Could you check a few things on this model? Use its own coordinates, in mm. A direction names the side the tool comes from. Give positions to 0.01 mm unless a question says otherwise; leave off trailing zeros. Loops run counter-clockwise (first coordinate to the right, second up) from the corner with the lowest first, then second, coordinate; pieces in that order, holes last. Notation, with made-up numbers: (75.25, -31) - (89.25, -31) arc R6 cw to (89.25, -23) - close; hole circle Ø9 at (48.25, 50). An arc over 180 degrees is marked (long way). Write each question's results on one line, items separated by ' | '. Start each with the question number.
```python
from build123d import *

# Parameters (mm, degrees)
SKETCH1_W           = 8.5
SKETCH1_H           = 8.5
BOSS_EXTRUDE1_DEPTH = 5
SKETCH2_W           = 8.5
SKETCH2_H           = 8.5
BOSS_EXTRUDE2_DEPTH = 2
SKETCH3_R           = 1.5
CUT_EXTRUDE1_DEPTH  = 2
SKETCH4_W           = 80
SKETCH4_H           = 8.5
BOSS_EXTRUDE3_DEPTH = 3
SKETCH5_W           = 7
SKETCH5_H           = 8.5
BOSS_EXTRUDE4_DEPTH = 8.5
CUT_EXTRUDE2_DEPTH  = 5
SKETCH7_R           = 1.5
CUT_EXTRUDE3_DEPTH  = 5
CUT_EXTRUDE4_DEPTH  = 10
SKETCH9_W           = 8.5
SKETCH9_H           = 8.5
SKETCH9_R           = 1.5
BOSS_EXTRUDE5_DEPTH = 2
CUT_EXTRUDE5_DEPTH  = 2
SKETCH11_W          = 8.5
SKETCH11_H          = 8.5
SKETCH11_R          = 1.5
BOSS_EXTRUDE6_DEPTH = 2
BOSS_EXTRUDE7_DEPTH = 5
BOSS_EXTRUDE8_DEPTH = 5
SKETCH14_W          = 8.5
SKETCH14_H          = 11.5
CUT_EXTRUDE6_DEPTH  = 4
SKETCH15_W          = 8.5
SKETCH15_H          = 11.5
CUT_EXTRUDE7_DEPTH  = 4
SKETCH16_R          = 1.5
CUT_EXTRUDE8_DEPTH  = 4
SKETCH17_R          = 1.5
CUT_EXTRUDE9_DEPTH  = 4


with BuildPart() as part:
    # Sketch1 → Boss-Extrude1 (new body)
    with BuildSketch(Plane(origin=(0, 0, 0), x_dir=(0, 0, -1), z_dir=(1, 0, 0))):
        Rectangle(SKETCH1_W, SKETCH1_H)
        Polygon((1.58771324, 2.75), (-1.58771324, 2.75), (-3.175426481, 0), (-1.58771324, -2.75), (1.58771324, -2.75), (3.175426481, 0), align=None, mode=Mode.SUBTRACT)
    extrude(amount=BOSS_EXTRUDE1_DEPTH)

    # Sketch2 → Boss-Extrude2 (add)
    with BuildSketch(Plane.ZY):
        Rectangle(SKETCH2_W, SKETCH2_H)
    extrude(amount=BOSS_EXTRUDE2_DEPTH)

    # Sketch3 → Cut-Extrude1 (cut)
    with BuildSketch(Plane(origin=(0, 0, 0), x_dir=(0, 0, -1), z_dir=(1, 0, 0))):
        Circle(SKETCH3_R)
    extrude(amount=-CUT_EXTRUDE1_DEPTH, mode=Mode.SUBTRACT)

    # Sketch4 → Boss-Extrude3 (add)
    with BuildSketch(Plane.XZ.offset(4.25)):
        with Locations((38, 0)):
            Rectangle(SKETCH4_W, SKETCH4_H)
    extrude(amount=BOSS_EXTRUDE3_DEPTH)

    # Sketch5 → Boss-Extrude4 (add)
    with BuildSketch(Plane(origin=(0, -4.25, 0), x_dir=(1, 0, 0), z_dir=(0, 1, 0))):
        with Locations((74.5, 0)):
            Rectangle(SKETCH5_W, SKETCH5_H)
    extrude(amount=BOSS_EXTRUDE4_DEPTH)

    # Sketch6 → Cut-Extrude2 (cut)
    with BuildSketch(Plane.ZY.offset(-71)):
        Polygon((3.175426481, 0), (1.58771324, 2.75), (-1.58771324, 2.75), (-3.175426481, 0), (-1.58771324, -2.75), (1.58771324, -2.75), align=None)
    extrude(amount=-CUT_EXTRUDE2_DEPTH, mode=Mode.SUBTRACT)

    # Sketch7 → Cut-Extrude3 (cut)
    with BuildSketch(Plane.ZY.offset(-76)):
        Circle(SKETCH7_R)
    extrude(amount=-CUT_EXTRUDE3_DEPTH, mode=Mode.SUBTRACT)

    # Sketch8 → Cut-Extrude4 (cut)
    with BuildSketch(Plane.ZY.offset(2)):
        Polygon((-1.58771324, 2.75), (1.58771324, 2.75), (3.175426481, 0), (1.58771324, -2.75), (-1.58771324, -2.75), (-3.175426481, 0), align=None)
    extrude(amount=-CUT_EXTRUDE4_DEPTH, mode=Mode.SUBTRACT)

    # Sketch9 → Boss-Extrude5 (add)
    with BuildSketch(Plane(origin=(5, 0, 0), x_dir=(0, 0, -1), z_dir=(1, 0, 0))):
        Rectangle(SKETCH9_W, SKETCH9_H)
        Circle(SKETCH9_R, mode=Mode.SUBTRACT)
    extrude(amount=-BOSS_EXTRUDE5_DEPTH)

    # Sketch10 → Cut-Extrude5 (cut)
    with BuildSketch(Plane(origin=(78, 0, 0), x_dir=(0, 0, -1), z_dir=(1, 0, 0))):
        Polygon((-3.175426481, 0), (-1.58771324, 2.75), (1.58771324, 2.75), (3.175426481, 0), (1.58771324, -2.75), (-1.58771324, -2.75), align=None)
    extrude(amount=-CUT_EXTRUDE5_DEPTH, mode=Mode.SUBTRACT)

    # Sketch11 → Boss-Extrude6 (add)
    with BuildSketch(Plane.ZY.offset(-71)):
        Rectangle(SKETCH11_W, SKETCH11_H)
        Circle(SKETCH11_R, mode=Mode.SUBTRACT)
    extrude(amount=-BOSS_EXTRUDE6_DEPTH)

    # Sketch12 → Boss-Extrude7 (add)
    with BuildSketch(Plane.ZY.offset(-3)):
        Polygon((-3.175426481, 0), (-1.58771324, 2.75), (1.58771324, 2.75), (3.175426481, 0), (1.58771324, -2.75), (-1.58771324, -2.75), align=None)
    extrude(amount=BOSS_EXTRUDE7_DEPTH)

    # Sketch13 → Boss-Extrude8 (add)
    with BuildSketch(Plane(origin=(73, 0, 0), x_dir=(0, 0, -1), z_dir=(1, 0, 0))):
        Polygon((-1.58771324, 2.75), (-3.175426481, 0), (-1.58771324, -2.75), (1.58771324, -2.75), (3.175426481, 0), (1.58771324, 2.75), align=None)
    extrude(amount=BOSS_EXTRUDE8_DEPTH)

    # Sketch14 → Cut-Extrude6 (cut)
    with BuildSketch(Plane.ZY.offset(2)):
        with Locations((0, -1.5)):
            Rectangle(SKETCH14_W, SKETCH14_H)
    extrude(amount=-CUT_EXTRUDE6_DEPTH, mode=Mode.SUBTRACT)

    # Sketch15 → Cut-Extrude7 (cut)
    with BuildSketch(Plane(origin=(78, 0, 0), x_dir=(0, 0, -1), z_dir=(1, 0, 0))):
        with Locations((0, -1.5)):
            Rectangle(SKETCH15_W, SKETCH15_H)
    extrude(amount=-CUT_EXTRUDE7_DEPTH, mode=Mode.SUBTRACT)

    # Sketch16 → Cut-Extrude8 (cut)
    with BuildSketch(Plane(origin=(5, 0, 0), x_dir=(0, 0, -1), z_dir=(1, 0, 0))):
        Circle(SKETCH16_R)
    extrude(amount=-CUT_EXTRUDE8_DEPTH, mode=Mode.SUBTRACT)

    # Sketch17 → Cut-Extrude9 (cut)
    with BuildSketch(Plane.ZY.offset(-73)):
        Circle(SKETCH17_R)
    extrude(amount=-CUT_EXTRUDE9_DEPTH, mode=Mode.SUBTRACT)


solid = part.part
```
Q1. I'm going to push flat-ended pins straight in: pin 1 Ø4 at (x, z) = (38.5, -1) entering from +Y; pin 2 Ø2.5 at (y, z) = (0, 0) entering from -X (1 decimal). Where does each tip first touch, or does it pass through?
Q2. I want a section at C-C, the plane z = 3. List the corners of the cut face in (x, y) for me.
Q3. I want a section at A-A, the plane y = 0. List the corners of the cut face in (x, z) for me, then the cut area to 3 significant figures.
Q4. If we mould it in two halves opening along X, with no side actions, what happens to faces 3 (the face through (38, -4.25, 0)), 4 (the face through (71, 0, -2)), 5 (the face through (4, 4.25, 0)), 6 (the face through (2, -1.4, -1))? For each: +X half, -X half, draft (parallel to the pull), parting line (faces both ways), or undercut.
Q5. Which directions (+Z, -Z, +X, -X, +Y, -Y) give clear straight access to the entire face, cutting with the end or side of a thin tool? Please do faces 1 (the face through (5, 0, -2)), 2 (the face through (72, 4.25, 0)).
Q6. I want a section at B-B, the plane z = 0. List the corners of the cut face in (x, y) for me, then the cut area to 3 significant figures.
Q7. I need wall thicknesses on L1, parallel to Y at x = 72.5, z = 0; L2, parallel to X at y = 2.5, z = 2; L3, parallel to Y at x = 27.5, z = 1.5. Which ranges of each line are inside material? Lowest first, please. Write a range as from..to.
Q8. I want a section at D-D, the plane x = 60.5. List the corners of the cut face in (y, z) for me, then the cut area to 3 significant figures.
Conclusion:
1) pin 1: y = -4.25 | pin 2: through
2) outline: (2, -7.25) - (74, -7.25) - (74, 4.25) - (71, 4.25) - (71, -4.25) - (5, -4.25) - (5, 4.25) - (2, 4.25) - close
3) outline: (2, -4.25) - (5, -4.25) - (5, -1.5) - (2, -1.5) - close; (2, 1.5) - (5, 1.5) - (5, 4.25) - (2, 4.25) - close; (71, -4.25) - (74, -4.25) - (74, -1.5) - (71, -1.5) - close; (71, 1.5) - (74, 1.5) - (74, 4.25) - (71, 4.25) - close | area: 33.0 mm^2
4) face 3: undercut | face 4: undercut | face 5: draft | face 6: -X half
5) face 1: +Z, -Z, +Y | face 2: +Z, -Z, +X, -X, +Y
6) outline: (2, -7.25) - (74, -7.25) - (74, -1.5) - (71, -1.5) - (71, -4.25) - (5, -4.25) - (5, -1.5) - (2, -1.5) - close; (2, 1.5) - (5, 1.5) - (5, 4.25) - (2, 4.25) - close; (71, 1.5) - (74, 1.5) - (74, 4.25) - (71, 4.25) - close | area: 249 mm^2
7) L1: -7.25..-1.5, 1.5..4.25 | L2: 2..5, 71..74 | L3: -7.25..-4.25
8) outline: (-7.25, -4.25) - (-4.25, -4.25) - (-4.25, 4.25) - (-7.25, 4.25) - close | area: 25.5 mm^2
